The listing builds one solid part. Answer for the finished solid, in the listing's coordinates (mm). Round coordinates to 2 decimals unless told otherwise and drop trailing zeros. Write each loop counter-clockwise with the first axis right and the second up, starting at its lowest first coordinate (ties: lowest second). Pieces come first, ordered by that corner, then holes.
(1) A cutting plane is placed at D-D, the plane x = 3.25. Give the vertices of the cut face in (y, z).
(2) Find the intervals of material crossed by probe 1 along Y at (x, z) = (-0.25, 0.2); probe 2 along X at (y, z) = (6, 0.2); probe 3 along X at (y, z) = (1.5, 0.1), in increasing order.
(3) A cutting plane is placed at B-B, the plane z = 0.1. Give the vertices of the cut face in (x, y), and give its area (3 significant figures).
(4) A cutting plane is placed at C-C, the plane x = -1. Give the vertices of the cut face in (y, z).
(5) A cutting plane is placed at A-A, the plane y = 6. Give the vertices of the cut face in (x, z).
Autodesk Inventor part; units mm, degrees
ref_plane "YZ Plane" through (0, 0, 0) normal (1, 0, 0) x (0, 1, 0)
ref_plane "XZ Plane" through (0, 0, 0) normal (0, 1, 0) x (-1, 0, 0)
ref_plane "XY Plane" through (0, 0, 0) normal (0, 0, 1) x (1, 0, 0)
sketch "Sketch1" plane through (0, 0, 0) normal (0, 0, 1) x (1, 0, 0)
  line L0 (-2.75, 3.25) -> (-4.7407, 3.4125)
  arc A0 (-5.2, 3.9108) -> (-4.7407, 3.4125) centre (-4.7, 3.9108) ccw
  line L1 (-5.2, 3.9108) -> (-5.2, 7.45)
  arc A1 (-4.7, 7.95) -> (-5.2, 7.45) centre (-4.7, 7.45) ccw
  arc A2 (5.2176, 3.2181) -> (5.6, 3.45) centre (5.1769, 3.7165) ccw
  line L2 (5.6, 3.45) -> (5.6, 7.75)
  arc A3 (5.6, 7.75) -> (5.1, 8.25) centre (5.1, 7.75) ccw
  line L3 (-5.1, 8.25) -> (5.1, 8.25)
  arc A4 (-5.1, 8.25) -> (-5.6, 7.75) centre (-5.1, 7.75) ccw
  line L4 (-5.6, 3.45) -> (-5.6, 7.75)
  arc A5 (-5.6, 3.45) -> (-5.2176, 3.2181) centre (-5.1769, 3.7165) ccw
  line L5 (-5.2176, 3.2181) -> (-3.1663, 3.0507)
  arc A6 (-3.15, 2.7961) -> (-3.1663, 3.0507) centre (-5.15, 2.7961) ccw
  line L6 (-3.15, -0.45) -> (-3.15, 2.7961)
  line L7 (3.15, -0.45) -> (-3.15, -0.45)
  line L8 (3.15, 2.7961) -> (3.15, -0.45)
  arc A7 (3.1663, 3.0507) -> (3.15, 2.7961) centre (5.15, 2.7961) ccw
  line L9 (3.1663, 3.0507) -> (5.2176, 3.2181)
  line L10 (2.75, -0.15) -> (2.75, 3.25)
  line L11 (-2.75, -0.15) -> (2.75, -0.15)
  line L12 (-2.75, 3.25) -> (-2.75, -0.15)
  line L13 (-2.75, 3.25) -> (-4.7407, 3.4125)
  arc A8 (-5.2, 3.9108) -> (-4.7407, 3.4125) centre (-4.7, 3.9108) ccw
  line L14 (-5.2, 3.9108) -> (-5.2, 7.45)
  arc A9 (-4.7, 7.95) -> (-5.2, 7.45) centre (-4.7, 7.45) ccw
  line L15 (-4.7, 7.95) -> (4.7, 7.95)
  arc A10 (5.2, 7.45) -> (4.7, 7.95) centre (4.7, 7.45) ccw
  line L16 (5.2, 3.9108) -> (5.2, 7.45)
  arc A11 (4.7407, 3.4125) -> (5.2, 3.9108) centre (4.7, 3.9108) ccw
  line L17 (4.7407, 3.4125) -> (2.75, 3.25)
  line L18 (-2.65, -0.05) -> (-2.65, 3.3422)
  line L19 (-2.65, 3.3422) -> (-4.7325, 3.5122)
  line L20 (-5.1, 3.9108) -> (-5.1, 7.45)
  line L21 (-4.7, 7.85) -> (4.7, 7.85)
  line L22 (5.1, 7.45) -> (5.1, 3.9108)
  line L23 (4.7325, 3.5122) -> (2.65, 3.3422)
  line L24 (2.65, 3.3422) -> (2.65, -0.05)
  line L25 (2.65, -0.05) -> (-2.65, -0.05)
  arc A12 (-5.1, 3.9108) -> (-4.7325, 3.5122) centre (-4.7, 3.9108) ccw
  arc A13 (4.7325, 3.5122) -> (5.1, 3.9108) centre (4.7, 3.9108) ccw
  arc A14 (-4.7, 7.85) -> (-5.1, 7.45) centre (-4.7, 7.45) ccw
  arc A15 (5.1, 7.45) -> (4.7, 7.85) centre (4.7, 7.45) ccw
  point P0 (0, 0)
  dimension "d0" = 0.1
  dimension "d1" = 0.1
  dimension "d2" = 0.1
  dimension "d3" = 0.1
  dimension "d4" = 0.1
  dimension "d5" = 0.1
  dimension "d6" = 0.1
  dimension "d7" = 0.1
  dimension "d8" = 0.4
  dimension "d9" = 0.4
  dimension "d10" = 0.4
  dimension "d11" = 0.4
extrude "Extrusion1" add sketch "Sketch1" along normal blind 0.3 contours L18 L19 A12 L20 A14 L21 A15 L22 A13 L23 L24 L25
sketch "Sketch2" plane through (0, 0, 0.3) normal (0, 0, 1) x (1, 0, 0)
  line L0 (-2.35, 6.8) -> (0.15, 6.8)
  line L1 (0.15, 6.8) -> (0.15, 4.3)
  line L2 (0.15, 4.3) -> (-2.35, 4.3)
  line L3 (-2.35, 4.3) -> (-2.35, 6.8)
  line L4 (-5.1, 7.45) -> (-5.1, 3.9108)
  line L5 (4.7, 7.85) -> (-4.7, 7.85)
  point P0 (0, 0)
  dimension "d14" = 2.75
  dimension "d15" = 1.05
  dimension "d16" = 2.5
  dimension "d17" = 2.5
extrude "Extrusion2" cut sketch "Sketch2" against normal blind 0.3
equation "\"d1\" = d0"
equation "\"d2\" = d0"
equation "\"d3\" = d0"
equation "\"d4\" = d0"
equation "\"d5\" = d0"
equation "\"d6\" = d0"
equation "\"d7\" = d0"
equation "\"d8\" = d10"
equation "\"d9\" = d10"
equation "\"d11\" = d10"
equation "\"d17\" = d16"
properties part number "top_enclosure"
Solutions:
1. outline: (3.39, 0) - (7.85, 0) - (7.85, 0.3) - (3.39, 0.3) - close
2. probe 1: y = -0.05 to 4.3, 6.8 to 7.85
2. probe 2: x = -5.1 to -2.35, 0.15 to 5.1
2. probe 3: x = -2.65 to 2.65
3. outline: (-5.1, 3.91) arc R0.4 ccw to (-4.73, 3.51) - (-2.65, 3.34) - (-2.65, -0.05) - (2.65, -0.05) - (2.65, 3.34) - (4.73, 3.51) arc R0.4 ccw to (5.1, 3.91) - (5.1, 7.45) arc R0.4 ccw to (4.7, 7.85) - (-4.7, 7.85) arc R0.4 ccw to (-5.1, 7.45) - close; hole (-2.35, 4.3) - (0.15, 4.3) - (0.15, 6.8) - (-2.35, 6.8) - close
3. area: 57.1 mm2
4. outline: (-0.05, 0) - (4.3, 0) - (4.3, 0.3) - (-0.05, 0.3) - close; (6.8, 0) - (7.85, 0) - (7.85, 0.3) - (6.8, 0.3) - close
5. outline: (-5.1, 0) - (-2.35, 0) - (-2.35, 0.3) - (-5.1, 0.3) - close; (0.15, 0) - (5.1, 0) - (5.1, 0.3) - (0.15, 0.3) - close
